For this review, take the finished solid that the model builds, in its own axes (mm). Face numbers are marked on the shaded views. A direction names the side the tool comes from. Round coordinates to 2 decimals unless told otherwise and drop trailing zeros. Answer in a Markdown table with one row per item.
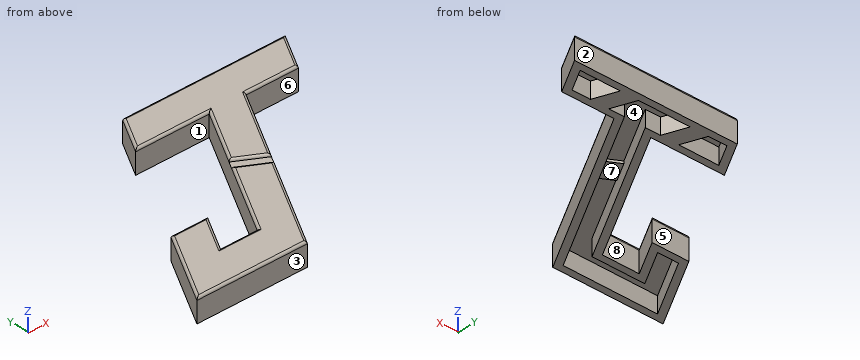
```python
from build123d import *

# Parameters (mm, degrees)
F1_DEPTH = 2.5
F4_W     = 1
F4_H     = 5.3799478337
F5_DEPTH = 100
F6_T     = -0.75
F7_R     = 0.24999
F9_DEPTH = 1.75


# Not quite as in the source:
# - a fillet or chamfer is up to 0.001 mm smaller than in the source, because OpenCascade refuses the exact size


with BuildPart() as f1:
    # F0 (on Top) → F1 (new body)
    with BuildSketch(Plane.XY):
        Polygon((-7.6905989232, 19), (-10, 15), (-2, 15), (-10.6602540378, 0), (-14.6602540378, 0), (-12.3508529611, 4), (-16.3508529611, 4), (-20.9696551146, -4), (-8.9696551146, -4), (2, 15), (7.6905989232, 15), (10, 19), align=None)
    extrude(amount=F1_DEPTH)

    # F4 (on offset) → F5 (cut)
    with BuildSketch(Plane(origin=(16.6554445662, -9.6160254038, 0), x_dir=(0.5, 0.8660254038, 0), z_dir=(0.8660254038, -0.5, 0))):
        with Locations((4.397114317, 4.9399739169)):
            Rectangle(F4_W, F4_H)
    extrude(amount=-F5_DEPTH, mode=Mode.SUBTRACT)

    # F6
    f6_openings = [f1.faces().sort_by_distance(p)[0] for p in [
        (-8.51122, 16.807119, 0),
    ]]
    offset(amount=F6_T, openings=f6_openings, kind=Kind.INTERSECTION)

    # F7 (radius 0.25 in the source; OpenCascade refuses exactly that, so slightly less here)
    f7_edges = [f1.edges().sort_by_distance(p)[0] for p in [
        (-0.273317, 11.0625, 2.5),
        (4.845299, 15, 2.5),
        (8.845299, 17, 2.5),
        (1.154701, 19, 2.5),
        (-8.845299, 17, 2.5),
        (-6, 15, 2.5),
        (-3.773317, 11.928525, 2.5),
        (-4.046633, 7.991025, 2.5),
        (-8.353444, 3.995513, 2.5),
        (-12.660254, 0, 2.5),
        (-13.505553, 2, 2.5),
        (-14.350853, 4, 2.5),
        (-18.660254, 0, 2.5),
        (-14.969655, -4, 2.5),
        (-6.008144, 1.129487, 2.5),
        (-4.546633, 7.125, 2.5),
    ]]
    fillet(f7_edges, radius=F7_R)

    # F8 (on face) → F9 (join, through all)
    with BuildSketch(Plane(origin=(0, 0, 1.75), x_dir=(1, 0, 0), z_dir=(0, 0, -1))):
        Polygon((-4.3476606357, -15.75), (-5.2575862213, -18.25), (-3.2575862213, -18.25), (-2.3476606357, -15.75), align=None)
        Polygon((3.2575862213, -15.75), (2.3476606357, -18.25), (4.3476606357, -18.25), (5.2575862213, -15.75), align=None)
    extrude(amount=F9_DEPTH)


solid = f1.part
```
Q1. Take a section at A-A, the plane z = 0.55. Give the number of separate pieces and of enclosed holes in the cut face, then the cut area to 3 significant figures.
Answer key:
| item | result |
|---|---|
| separate pieces | 1 |
| enclosed holes | 3 |
| area | 92.7 mm^2 |
Q2. Clearance check with flat-ended pins moving along their axes: pin 1 Ø1.1 at (x, z) = (5.5, 1.5) entering from -Y; pin 2 Ø0.8 at (x, y) = (-6, 16.5) entering from -Z; pin 3 Ø1.4 at (x, z) = (-16.5, 0.5) entering from +Y. State where each tip first meets the part, or that it passes through.
Answer key:
| item | result |
|---|---|
| pin 1 | stops at y = 15 |
| pin 2 | stops at z = 1.75 |
| pin 3 | stops at y = 4 |
Q3. The part is to be moulded in two halves that separate along Y. For the marked faces 1, 2, 3 and 4, say which applies: +Y half, -Y half, draft (parallel to the pull), parting line (faces both ways), or undercut.
Answer key:
| item | result |
|---|---|
| face 1 | undercut |
| face 2 | +Y half |
| face 3 | -Y half |
| face 4 | undercut |
Q4. Tool access review of the marked faces 5, 6, 7 and 8: name each direction out of +Z, -Z, +X, -X, +Y, -Y from which nothing blocks a thin tool from reaching the whole face with its end or side.
Answer key:
| item | result |
|---|---|
| face 5 | +Z, -Z, -X, +Y |
| face 6 | +Z, -Z, +X, -Y |
| face 7 | -Z |
| face 8 | +Z, -Z |
Q5. To check wall thickness, follow probe 1 along Y at (x, z) = (-16.5, 1.25); probe 2 along Y at (x, z) = (-13, 1); probe 3 along Y at (x, z) = (6.5, 1.15). State the ranges of each line that lie inside material, in increasing order.
Answer key:
| item | result |
|---|---|
| probe 1 | y = -4 to -3.25, 2.24 to 3.74 |
| probe 2 | y = -4 to -3.25, -0.75 to 0, 2.88 to 4 |
| probe 3 | y = 15 to 15.75, 18.25 to 19 |
